Geometry check sheet. Reference: the model listing, model coordinates, mm. A direction names the side the tool comes from. Round coordinates to 2 decimals unless told otherwise and drop trailing zeros. Order: outer loops, then holes, each group sorted by start corner. A loop starts at its lowest first (then second) coordinate and runs counter-clockwise, first axis right, second up.
(1) Sectioned sample at C-C (y = -0.35). Record the boundary of the cut face in (x, z), plus the area to 3 significant figures.
(2) Go/stop test with flat-tipped pins: pin 1 (0.6 mm diameter, centred on x = 1.5, z = -2, fed in from +Y); pin 2 (3 mm diameter, centred on x = 3, z = 5.5, fed in from +Y); pin 3 (0.9 mm diameter, centred on y = 0.5, z = -0.5, fed in from +X). Record where each tip stops, or that it passes through.
(3) Set-up check for faces 4 (the face through (3.54, -0.78, 5.17)), 5 (the face through (1.14, 0.6, -0.1)): record each of +Z, -Z, +X, -X, +Y, -Y from which the full face is reachable in a straight line by a thin tool's end or side.
(4) Sectioned sample at D-D (x = 2.8). Record the boundary of the cut face in (y, z), plus the area to 3 significant figures.
(5) Material ranges on line 1 along Z through (x, y) = (2.2, -0.35); line 2 along Y through (x, z) = (0, 7.6); line 3 along Y through (x, z) = (0.2, -2), recorded low to high.
(6) Release check for a two-part mould opening along X. For faces 1 (the face through (-0.44, 1.89, 5.17)), 2 (the face through (3.26, 1.85, 5.17)), 3 (the face through (1.64, 0.6, -0.1)) record: +X half, -X half, draft (parallel to the pull), parting line (faces both ways), or undercut.
(7) Sectioned sample at A-A (x = 0). Record the boundary of the cut face in (y, z), plus the area to 3 significant figures.
(8) Sectioned sample at B-B (z = 0.25). Give the number of separate pieces and of enclosed holes in the cut face, plus the area to 3 significant figures.
from build123d import *

# Parameters (mm, degrees)
EXTRUDE_1_DEPTH          = 5.33
SKETCH_1_W               = 0.5
SKETCH_1_H               = 0.5
EXTRUDE_2_DEPTH          = 2.54
SKETCH_1_2_W             = 0.5
SKETCH_1_2_H             = 0.5
EXTRUDE_3_DEPTH          = 10.16
SKETCH_4_R               = 0.2
CUT_EXTRUDE_1_DEPTH      = 0.5
SKETCH_5_W               = 0.5
SKETCH_5_H               = 10.2
EXTRUDE_4_DEPTH          = 1.25
CUT_EXTRUDE_2_DEPTH      = 10
CUT_EXTRUDE_2_DEPTH_BACK = 10
FILLET_1_R               = 0.5
FILLET_2_R               = 1
SKETCH_7_W               = 0.5
SKETCH_7_H               = 0.75
CUT_EXTRUDE_3_DEPTH      = 2
FILLET_3_R               = 1


with BuildPart() as part:
    # Эскиз3 → Вытянуть1 (new body)
    with BuildSketch(Plane.XY.offset(2.54)):
        with BuildLine():
            Line((-0.325, -1.53), (3.105, -1.53))
            Line((3.105, -1.53), (3.99, 0))
            ThreePointArc((3.99, 0), (3.240904038, 1.868477631), (1.39, 2.66))
            ThreePointArc((1.39, 2.66), (-0.460904038, 1.868477631), (-1.21, 0))
            Line((-1.21, 0), (-0.325, -1.53))
        make_face()
    extrude(amount=EXTRUDE_1_DEPTH)

    # Эскиз1 → Вытянуть2 (add)
    with BuildSketch(Plane.XY):
        with Locations((1.39, 0)):
            Rectangle(SKETCH_1_W, SKETCH_1_H)
        Rectangle(SKETCH_1_W, SKETCH_1_H)
        with Locations((2.78, 0)):
            Rectangle(SKETCH_1_W, SKETCH_1_H)
    extrude(amount=EXTRUDE_2_DEPTH)

    # Эскиз1<2> → Вытянуть3 (add)
    with BuildSketch(Plane.XY):
        with Locations((1.39, 0)):
            Rectangle(SKETCH_1_2_W, SKETCH_1_2_H)
        Rectangle(SKETCH_1_2_W, SKETCH_1_2_H)
        with Locations((2.78, 0)):
            Rectangle(SKETCH_1_2_W, SKETCH_1_2_H)
    extrude(amount=-EXTRUDE_3_DEPTH)

    # Эскиз4 → Вырез-Вытянуть1 (cut)
    with BuildSketch(Plane.XY.offset(7.87)):
        Circle(SKETCH_4_R)
    extrude(amount=-CUT_EXTRUDE_1_DEPTH, mode=Mode.SUBTRACT)

    # Эскиз5 → Вытянуть4 (add)
    with BuildSketch(Plane(origin=(0, 0.25, 0), x_dir=(1, 0, 0), z_dir=(0, 1, 0))):
        with Locations((1.39, 5.06)):
            Rectangle(SKETCH_5_W, SKETCH_5_H)
    extrude(amount=EXTRUDE_4_DEPTH)

    # Эскиз6 → Вырез-Вытянуть2 (cut, two sides: drawn at the far end of the back side and taken through both)
    with BuildSketch(Plane(origin=(1.64, 0, 0), x_dir=(0, 0, -1), z_dir=(1, 0, 0)).offset(-CUT_EXTRUDE_2_DEPTH_BACK)):
        with BuildLine():
            Line((2.46, -0.83850211), (10.787068804, -0.83850211))
            Line((10.787068804, -0.83850211), (10.787068804, 1))
            Line((10.787068804, 1), (10.787068804, 2.286855948))
            Line((10.787068804, 2.286855948), (2.46, 2.286855948))
            Line((2.46, 2.286855948), (2.46, 1))
            Line((2.46, 1), (0.96, 1))
            ThreePointArc((0.96, 1), (0.606446609, 0.853553391), (0.46, 0.5))
            Line((0.46, 0.5), (2.46, 0.5))
            Line((2.46, 0.5), (2.46, -0.83850211))
        make_face()
    extrude(amount=CUT_EXTRUDE_2_DEPTH + CUT_EXTRUDE_2_DEPTH_BACK, mode=Mode.SUBTRACT)

    # Скругление1
    fillet_1_edges = [part.edges().sort_by_distance(p)[0] for p in [
        (1.39, 0.25, 0.04),
    ]]
    fillet(fillet_1_edges, radius=FILLET_1_R)

    # Скругление2
    fillet_2_edges = [part.edges().sort_by_distance(p)[0] for p in [
        (1.39, 1.5, 0.04),
    ]]
    fillet(fillet_2_edges, radius=FILLET_2_R)

    # Эскиз7 → Вырез-Вытянуть3 (cut)
    with BuildSketch(Plane(origin=(0, 0, -2.46), x_dir=(-1, 0, 0), z_dir=(0, 0, -1))):
        with Locations((-1.39, 0.125)):
            Rectangle(SKETCH_7_W, SKETCH_7_H)
    extrude(amount=-CUT_EXTRUDE_3_DEPTH, mode=Mode.SUBTRACT)

    # Скругление3
    fillet_3_edges = [part.edges().sort_by_distance(p)[0] for p in [
        (1.39, -0.25, -0.46),
    ]]
    fillet(fillet_3_edges, radius=FILLET_3_R)


solid = part.part
Answer below:
1. outline: (-1.01, 2.54) - (3.79, 2.54) - (3.79, 7.87) - (-1.01, 7.87) - close
1. area: 25.6 mm2
2. pin 1: stops at y = 1.5
2. pin 2: stops at y = 2.66
2. pin 3: stops at x = 3.03
3. face 4: +Z, -Z, +X, -Y
3. face 5: -Z, +Y, -Y
4. outline: (-1.53, 2.54) - (-0.25, 2.54) - (-0.25, -2.46) - (0.25, -2.46) - (0.25, 2.54) - (2.23, 2.54) - (2.23, 7.87) - (-1.53, 7.87) - close
4. area: 22.5 mm2
5. line 1: z = 2.54 to 7.87
5. line 2: y = -1.53 to -0.2, 0.2 to 2.24
5. line 3: y = -0.25 to 0.25
6. face 1: -X half
6. face 2: +X half
6. face 3: undercut
7. outline: (-1.53, 2.54) - (-0.25, 2.54) - (-0.25, -2.46) - (0.25, -2.46) - (0.25, 2.54) - (2.24, 2.54) - (2.24, 7.87) - (0.2, 7.87) - (0.2, 7.37) - (-0.2, 7.37) - (-0.2, 7.87) - (-1.53, 7.87) - close
7. area: 22.4 mm2
8. separate pieces: 3
8. enclosed holes: 0
8. area: 0.778 mm2
